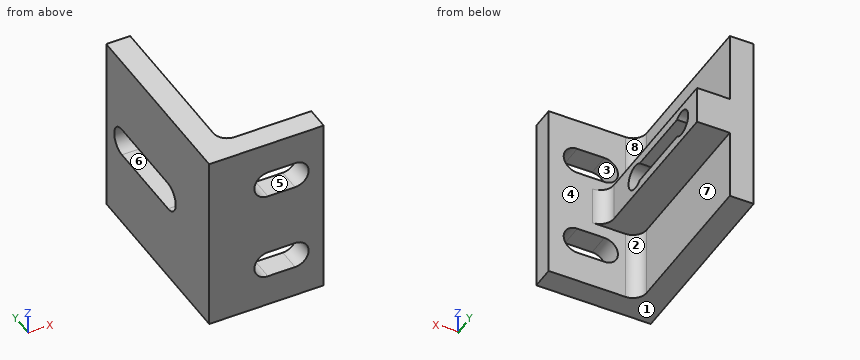
from build123d import *

# Parameters (mm, degrees)
EXTRUDE_THIN1_DEPTH     = 30
EXTRUDE5_DEPTH          = 4.81
SKETCH10_W              = 5.588
SKETCH10_H              = 27.94
BOSS_EXTRUDE1_DEPTH     = 30
CUT_EXTRUDE1_DEPTH      = 16.19
CUT_EXTRUDE1_DEPTH_BACK = 4.81
F_8_32_TAPPED_HOLE1_D   = 4.1656
SKETCH14_W              = 5.4356
SKETCH14_H              = 11.825
CUT_EXTRUDE2_DEPTH      = 27.94
FILLET1_R               = 2.286
FILLET2_R               = 2.286
CUT_EXTRUDE3_DEPTH      = 5.9944


with BuildPart() as part:
    # Sketch1 → Extrude-Thin1 (new body)
    with BuildSketch(Plane.XY):
        Polygon((0, 31.75), (0, 0), (19, 0), (19, 3.81), (3.81, 3.81), (3.81, 31.75), align=None)
    extrude(amount=-EXTRUDE_THIN1_DEPTH)

    # Sketch6 → Extrude5 (cut, through all)
    with BuildSketch(Plane(origin=(0, 3.81, 0), x_dir=(1, 0, 0), z_dir=(0, 1, 0))):
        with BuildLine():
            Line((14.2502, 24.75), (9.7502, 24.75))
            ThreePointArc((9.7502, 24.75), (7.5002, 22.5), (9.7502, 20.25))
            Line((9.7502, 20.25), (14.2502, 20.25))
            ThreePointArc((14.2502, 20.25), (16.5002, 22.5), (14.2502, 24.75))
        make_face()
        with BuildLine():
            Line((9.7502, 9.75), (14.2502, 9.75))
            ThreePointArc((14.2502, 9.75), (16.5002, 7.5), (14.2502, 5.25))
            Line((14.2502, 5.25), (9.7502, 5.25))
            ThreePointArc((9.7502, 5.25), (7.5002, 7.5), (9.7502, 9.75))
        make_face()
    extrude(amount=-EXTRUDE5_DEPTH, mode=Mode.SUBTRACT)

    # Sketch10 → Boss-Extrude1 (add)
    with BuildSketch(Plane.XY):
        with Locations((6.604, 17.78)):
            Rectangle(SKETCH10_W, SKETCH10_H)
    extrude(amount=-BOSS_EXTRUDE1_DEPTH)

    # Sketch4 → Cut-Extrude1 (cut, two sides)
    with BuildSketch(Plane(origin=(3.81, 0, 0), x_dir=(0, 0, -1), z_dir=(1, 0, 0))) as cut_extrude1_sk:
        with BuildLine():
            Line((13.4125, 12.7), (13.4125, 26.924))
            ThreePointArc((13.4125, 26.924), (15, 28.5115), (16.5875, 26.924))
            Line((16.5875, 26.924), (16.5875, 12.7))
            ThreePointArc((16.5875, 12.7), (15, 11.1125), (13.4125, 12.7))
        make_face()
    extrude(amount=CUT_EXTRUDE1_DEPTH, mode=Mode.SUBTRACT)
    extrude(cut_extrude1_sk.sketch, amount=-CUT_EXTRUDE1_DEPTH_BACK, mode=Mode.SUBTRACT)

    # #8-32 Tapped Hole1 (through all)
    with Locations(Plane(origin=(9.398, 0, 0), x_dir=(0, 0, -1), z_dir=(1, 0, 0))):
        with Locations((15, 12.7), (15, 26.924)):
            Hole(F_8_32_TAPPED_HOLE1_D / 2)

    # Sketch14 → Cut-Extrude2 (cut)
    with BuildSketch(Plane(origin=(0, 31.75, 0), x_dir=(1, 0, 0), z_dir=(0, 1, 0))):
        with Locations((6.6802, 24.0875)):
            Rectangle(SKETCH14_W, SKETCH14_H)
        with Locations((6.6802, 5.9125)):
            Rectangle(SKETCH14_W, SKETCH14_H)
    extrude(amount=-CUT_EXTRUDE2_DEPTH, mode=Mode.SUBTRACT)

    # Fillet1
    fillet1_edges = [part.edges().sort_by_distance(p)[0] for p in [
        (9.398, 3.81, -15),
    ]]
    fillet(fillet1_edges, radius=FILLET1_R)

    # Fillet2
    fillet2_edges = [part.edges().sort_by_distance(p)[0] for p in [
        (3.9624, 3.81, -24.0875),
        (3.9624, 3.81, -5.9125),
    ]]
    fillet(fillet2_edges, radius=FILLET2_R)

    # Sketch11 → Cut-Extrude3 (cut)
    with BuildSketch(Plane(origin=(0, 0, 5.175), x_dir=(0, 0, -1), z_dir=(1, 0, 0))):
        with BuildLine():
            Line((17.8001, 12.7), (17.8001, 26.924))
            ThreePointArc((17.8001, 26.924), (20.175, 29.2989), (22.5499, 26.924))
            Line((22.5499, 26.924), (22.5499, 12.7))
            ThreePointArc((22.5499, 12.7), (20.175, 10.3251), (17.8001, 12.7))
        make_face()
    extrude(amount=CUT_EXTRUDE3_DEPTH, mode=Mode.SUBTRACT)


solid = part.part
Check sheet for the modelled part. Datum: model origin and axes. Units: mm. Face numbers are marked on the shaded views. A direction names the side the tool comes from. Coordinates: 2 decimals unless noted, no trailing zeros. Loops run counter-clockwise (first coordinate to the right, second up) from the corner with the lowest first, then second, coordinate; pieces in that order, holes last. Notation, with made-up numbers: (64.25, -13) -> (104.25, -13) arc R10 ccw to (104.25, -8) -> close; hole circle Ø10 at (-31.75, -19). An arc over 180 degrees is marked (long way). Write item = value, one per line. Start each with the question number.
1. Tool access check on the marked faces 4, 5, 6, 7 and 8. Record the directions out of +Z, -Z, +X, -X, +Y, -Y that give a thin tool (end or side, any length) a straight path to the whole face; none if there is none.
2. Draft check along Z on the marked faces 1, 2 and 3. Enter one of: released by +Z, released by -Z, zero draft, split by the parting line, or undercut.
3. Material ranges on line 1 (Z direction, x = 7.75, y = 12.7) (3 decimals); line 2 (Z direction, x = 2, y = 22); line 3 (Y direction, x = 6.8, z = -15), recorded low to high.
4. Section check B-B on z = -22.5. Record the cut outline in (x, y).
5. Section check C-C on y = 7. Record the cut outline in (x, z) (3 decimals), then the cut area to 3 significant figures.
6. Section check A-A on y = 18. Record the cut outline in (x, z) (1 decimal), then the cut area to 3 significant figures.
7. Section check D-D on x = 15.5. Record the cut outline in (y, z).
8. Depth check by flat-ended pin: P1, Ø2.5, axis at x = 7, y = 18.5, coming from the -Z side (3 decimals); P2, Ø1.7, axis at x = 8, y = 22, coming from the +Z side (3 decimals); P3, Ø12, axis at y = 18, z = -25, coming from the +X side; P4, Ø2.5, axis at y = 16.5, z = -15, coming from the -X side. Enter the tip coordinate at first touch or a pass-through.
Responses:
q1.face_4 = +X, +Y
q1.face_5 = +Y, -Y
q1.face_6 = -X
q1.face_7 = -Z, +X, +Y
q1.face_8 = +Z, +X, +Y
q2.face_1 = released by -Z
q2.face_2 = zero draft
q2.face_3 = undercut
q3.line_1 = -18.175 to -17.083, -12.917 to -11.825
q3.line_2 = -30 to -17.37, -12.63 to 0
q3.line_3 = 0 to 10.62, 29.01 to 31.75
q4.outline = (0, 0) -> (7.5, 0) -> (7.5, 3.81) -> (6.25, 3.81) arc R2.29 cw to (3.96, 6.1) -> (3.96, 31.75) -> (0, 31.75) -> close; (16.5, 0) -> (19, 0) -> (19, 3.81) -> (16.5, 3.81) -> close
q5.outline = (0, -30) -> (3.962, -30) -> (3.962, -18.175) -> (9.398, -18.175) -> (9.398, -11.825) -> (3.962, -11.825) -> (3.962, 0) -> (0, 0) -> close
q5.area = 153 mm2
q6.outline = (0, -30) -> (4, -30) -> (4, -18.2) -> (9.4, -18.2) -> (9.4, -16.6) -> (6, -16.6) -> (6, -17.4) -> (0, -17.4) -> close; (0, -12.6) -> (6, -12.6) -> (6, -13.4) -> (9.4, -13.4) -> (9.4, -11.8) -> (4, -11.8) -> (4, 0) -> (0, 0) -> close
q6.area = 114 mm2
q7.outline = (0, -30) -> (3.81, -30) -> (3.81, -24.37) -> (0, -24.37) -> close; (0, -20.63) -> (3.81, -20.63) -> (3.81, -9.37) -> (0, -9.37) -> close; (0, -5.63) -> (3.81, -5.63) -> (3.81, 0) -> (0, 0) -> close
q8.P1 = -18.175
q8.P2 = -11.825
q8.P3 = 3.96
q8.P4 = through
